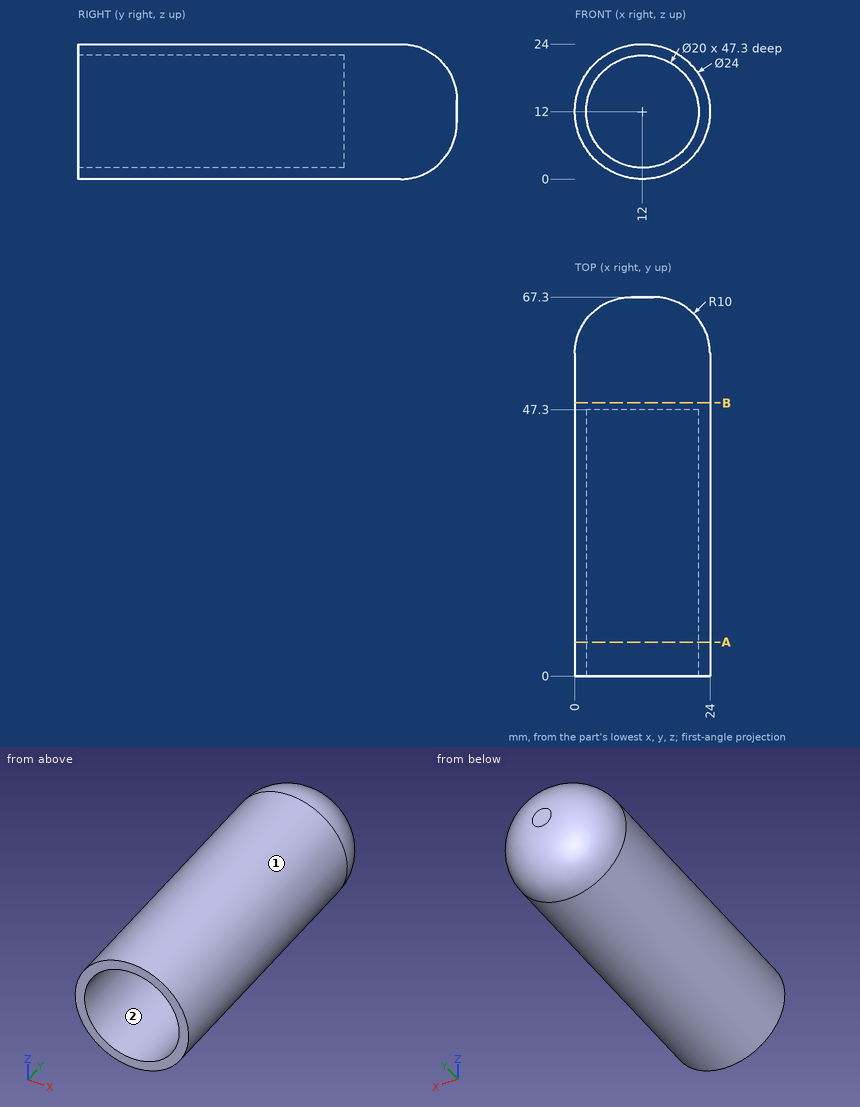
Input: dimensioned drawing with shaded views. Units: mm. Origin: part minimum x, y, z. Give positions to 0.01 mm unless a question says otherwise; leave off trailing zeros. Write each loop counter-clockwise with the first axis right and the second up, starting at its lowest first coordinate (ties: lowest second). Pieces come first, ordered by that corner, then holes.
1. Pull-direction query (Z, two-part tool) for the marked faces 1 and 2; classes: +Z half, -Z half, draft (parallel to the pull), parting line (faces both ways), or undercut.
2. Section query B-B (y = 48.5). Return the cut outline in (x, z), then the cut area to 3 significant figures.
3. Section query A-A (y = 6). Return the cut outline in (x, z).
4. First-contact query: pin 1 (1.5 mm diameter, centred on x = 8.5, z = 9, fed in from -Y); pin 2 (6 mm diameter, centred on y = 43, z = 7.5, fed in from +X); pin 3 (10 mm diameter, centred on x = 5.5, y = 43.5, fed in from +Z). Flat tips, straight axial feed; report the tip coordinate or a pass-through.
5. Material intervals for line 1 along X through (y, z) = (34.5, 12); line 2 along Z through (x, y) = (11.25, 15.5); line 3 along X through (y, z) = (41.5, 14.5), sorted ascending.
Output values:
1. face 1: parting line
1. face 2: undercut
2. outline: circle Ø24 at (12, 12)
2. area: 452 mm2
3. outline: circle Ø24 at (12, 12); hole circle Ø20 at (12, 12)
4. pin 1: stops at y = 47.3
4. pin 2: stops at x = 23.91
4. pin 3: stops at z = 23.91
5. line 1: x = 0 to 2, 22 to 24
5. line 2: z = 0.02 to 2.03, 21.97 to 23.98
5. line 3: x = 0.26 to 2.32, 21.68 to 23.74
